Can you work these out from the model? Positions are in its coordinate system, mm. A direction names the side the tool comes from. Coordinates: 2 decimals unless noted, no trailing zeros. Loops run counter-clockwise (first coordinate to the right, second up) from the corner with the lowest first, then second, coordinate; pieces in that order, holes last. Notation, with made-up numbers: (-21.5, -35.75) - (34.5, -35.75) arc R30 cw to (34.5, -10.75) - close; hole circle Ø8 at (46.25, 6.5). An arc over 180 degrees is marked (long way). Put each result on its own line as item: value. Start each with the question number.
from build123d import *

# Parameters (mm, degrees)
F0_W     = 336.55
F0_H     = 44.45
F1_DEPTH = 44.45
F2_W     = 508
F2_H     = 177.8
F3_DEPTH = 31.75
F6_DEPTH = 19.05


with BuildPart() as f1:
    # F0 (on Front) → F1 (new body)
    with BuildSketch(Plane.XZ):
        Rectangle(F0_W, F0_H)
        Polygon((-168.275, -22.225), (-168.275, 22.225), (-212.725, 22.225), (-212.725, -358.775), (-168.275, -358.775), align=None)
        Polygon((212.725, 22.225), (168.275, 22.225), (168.275, -22.225), (168.275, -358.775), (212.725, -358.775), align=None)
    extrude(amount=F1_DEPTH)

    # F2 (on face) → F3 (join)
    with BuildSketch(Plane.XY.offset(22.225)):
        with Locations((0, -63.5)):
            Rectangle(F2_W, F2_H)
    extrude(amount=F3_DEPTH)

    # F5 (on offset) → F6 (join)
    with BuildSketch(Plane(origin=(0, 0, -219.075), x_dir=(1, 0, 0), z_dir=(0, 0, -1))):
        Polygon((-168.275, 44.45), (-168.275, 25.4), (168.275, 25.4), (168.275, 44.45), (168.275, 152.6916772127), (-168.275, 152.6916772127), align=None)
    extrude(amount=F6_DEPTH)


solid = f1.part
Q1. I want a section at D-D on y = -32.5. List the corners of the cut face in (x, z) for me (3 decimals), and give its area (3 significant figures).
Q2. I want a section at B-B on z = -248.5. List the corners of the cut face in (x, y) for me (3 decimals), and give its area (3 significant figures).
Q3. We'd pull the mould along Z, two halves only. Please class faces 5 (the flat face through (-17, -44.45, -12)), 6 (the flat face through (-191, -22, -358.775)), 7 (the flat face through (168.275, -98, -228)): released by +Z, released by -Z, zero draft, split by the parting line, or undercut.
Q4. Will these pins go through, and if not, where does the flat tip stop? pin 1 (5.5 mm diameter, centred on x = -68.5, z = -227, fed in from +Y); pin 2 (21 mm diameter, centred on y = -86, z = -230, fed in from -X) (3 decimals); pin 3 (9.5 mm diameter, centred on x = 84.5, z = 36, fed in from -Y).
Q5. On a 3-axis mill with a long thin cutter (end or side, diameter ignored), from which of +Z, -Z, +X, -X, +Y, -Y can I reach the whole of each face in a straight line? I mean faces 1 (the flat face through (-17, 0, -12)), 2 (the flat face through (-2, -22, -22.225)), 3 (the flat face through (-2, -25.4, -228)), 4 (the flat face through (212.725, -22, -171)). Say none if no direction works.
Q6. I want a section at A-A on y = -117.5. List the corners of the cut face in (x, z) for me (3 decimals), and give its area (3 significant figures).
Q7. I want a section at C-C on x = 20. List the corners of the cut face in (y, z) for me (3 decimals).
Q8. Please list where these lines run through material, in increasing order: line 1 along Z through (x, y) = (-130, -95) (3 decimals); line 2 along Z through (x, y) = (-49, -29.5) (3 decimals); line 3 along X through (y, z) = (-30, -246) (3 decimals). Write a range as [from, to].
Calculated:
1. outline: (-254, 22.225) - (-212.725, 22.225) - (-212.725, -358.775) - (-168.275, -358.775) - (-168.275, -238.125) - (168.275, -238.125) - (168.275, -358.775) - (212.725, -358.775) - (212.725, 22.225) - (254, 22.225) - (254, 53.975) - (-254, 53.975) - close; hole (-168.275, -219.075) - (168.275, -219.075) - (168.275, -22.225) - (-168.275, -22.225) - close
1. area: 71,400 mm2
2. outline: (-212.725, -44.45) - (-168.275, -44.45) - (-168.275, 0) - (-212.725, 0) - close; (168.275, -44.45) - (212.725, -44.45) - (212.725, 0) - (168.275, 0) - close
2. area: 3,950 mm2
3. face 5: undercut
3. face 6: released by -Z
3. face 7: zero draft
4. pin 1: y = -25.4
4. pin 2: x = -168.275
4. pin 3: y = -152.4
5. face 1: -Z, +X, -X, +Y
5. face 2: +Y, -Y
5. face 3: -Z, +Y
5. face 4: -Z, +X, +Y, -Y
6. outline: (-254, 22.225) - (254, 22.225) - (254, 53.975) - (-254, 53.975) - close; (-168.275, -238.125) - (168.275, -238.125) - (168.275, -219.075) - (-168.275, -219.075) - close
6. area: 22,500 mm2
7. outline: (-152.692, -238.125) - (-25.4, -238.125) - (-25.4, -219.075) - (-152.692, -219.075) - close; (-152.4, 22.225) - (-44.45, 22.225) - (-44.45, -22.225) - (0, -22.225) - (0, 22.225) - (25.4, 22.225) - (25.4, 53.975) - (-152.4, 53.975) - close
8. line 1: [-238.125, -219.075], [22.225, 53.975]
8. line 2: [-238.125, -219.075], [-22.225, 53.975]
8. line 3: [-212.725, -168.275], [168.275, 212.725]
